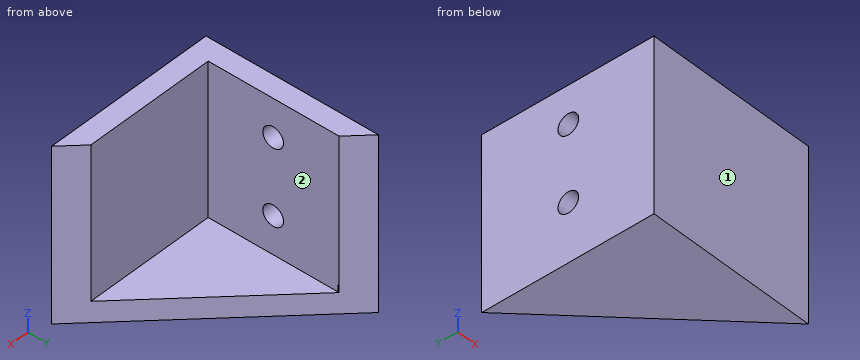
from build123d import *

# Parameters (mm, degrees)
BOSS_EXTRUDE2_DEPTH     = 25
CUT_EXTRUDE1_DEPTH      = 21
SKETCH3_W               = 26.870057685
SKETCH3_H               = 1
CUT_EXTRUDE3_DEPTH      = 0.1
CUT_EXTRUDE4_DEPTH      = 1
BOSS_EXTRUDE3_DEPTH     = 1
CUT_EXTRUDE5_DEPTH      = 15
CUT_EXTRUDE5_DEPTH_BACK = 18
SKETCH8_R               = 1.5


with BuildPart() as part:
    # Sketch1 → Boss-Extrude2 (new body)
    with BuildSketch(Plane.XY):
        Polygon((0, 24.307463671), (0, -0.692536329), (25, -0.692536329), align=None)
    extrude(amount=BOSS_EXTRUDE2_DEPTH)

    # Sketch2 → Cut-Extrude1 (cut)
    with BuildSketch(Plane.XY.offset(25)):
        Polygon((3, 21.307463671), (3, 2.307463671), (22, 2.307463671), align=None)
    extrude(amount=-CUT_EXTRUDE1_DEPTH, mode=Mode.SUBTRACT)

    # Sketch3 → Cut-Extrude3 (cut)
    with BuildSketch(Plane(origin=(12.153731836, 12.153731836, 0), x_dir=(0.7071067811865475, -0.7071067811865477, 0), z_dir=(0.7071067811865477, 0.7071067811865475, 0))):
        with Locations((0.489697135, -3.5)):
            Rectangle(SKETCH3_W, SKETCH3_H)
    extrude(amount=-CUT_EXTRUDE3_DEPTH, mode=Mode.SUBTRACT)

    # Sketch4 → Cut-Extrude4 (cut)
    with BuildSketch(Plane.XY.offset(4)):
        Polygon((3, 21.307463671), (3, 2.307463671), (22, 2.307463671), align=None)
    extrude(amount=-CUT_EXTRUDE4_DEPTH, mode=Mode.SUBTRACT)

    # Sketch5 → Boss-Extrude3 (add)
    with BuildSketch(Plane.XY.offset(3)):
        Polygon((22, 2.307463671), (21.858578644, 2.307463671), (21.929289322, 2.236752993), align=None)
    extrude(amount=BOSS_EXTRUDE3_DEPTH)

    # Sketch8 → Cut-Extrude5 (cut, two sides: drawn at the far end of the back side and taken through both)
    with BuildSketch(Plane(origin=(3, 0, 0), x_dir=(0, 0, -1), z_dir=(1, 0, 0)).offset(-CUT_EXTRUDE5_DEPTH_BACK)):
        with Locations(Location((-8.5, 11.736752993, 0), (0, 0, 270))):
            Circle(SKETCH8_R)
        with Locations(Location((-19.5, 11.736752993, 0), (0, 0, 270))):
            Circle(SKETCH8_R)
    extrude(amount=CUT_EXTRUDE5_DEPTH + CUT_EXTRUDE5_DEPTH_BACK, mode=Mode.SUBTRACT)


solid = part.part
Can you work these out from the model? Positions are in its coordinate system, mm. Face numbers are marked on the shaded views. A direction names the side the tool comes from. Give positions to 0.01 mm unless a question says otherwise; leave off trailing zeros. Loops run counter-clockwise (first coordinate to the right, second up) from the corner with the lowest first, then second, coordinate; pieces in that order, holes last. Notation, with made-up numbers: M 25.25,15 L 79.25,15 A27 cw 79.25,44 Z; hole C -1,79 d8. An arc over 180 degrees is marked long. One line per item, written item: value. Start each with the question number.
1) If we section it at A-A, the plane z = 8.5: Write out the boundary of the cut face in (x, y), and give its area (3 significant figures).
2) On a 3-axis mill with a long thin cutter (end or side, diameter ignored), from which of +Z, -Z, +X, -X, +Y, -Y can I reach the whole of each face in a straight line? I mean the marked faces 1 and 2. Say none if no direction works.
3) If we section it at C-C, the plane x = 15.5: Write out the boundary of the cut face in (y, z), and give its area (3 significant figures).
4) If we section it at B-B, the plane z = 15.75: Write out the boundary of the cut face in (x, y).
5) If I drill on line 1 (Y direction, x = 19, z = 6.5); line 2 (X direction, y = 16.25, z = 12.25), over which ranges is the centre line in solid material (lowest first)? Write a range as [from, to].
6) I'm going to push flat-ended pins straight in: pin 1 (6 mm diameter, centred on y = 7.5, z = 4, fed in from -X); pin 2 (5 mm diameter, centred on x = 11.5, z = 18.5, fed in from +Y); pin 3 (15 mm diameter, centred on y = 10, z = 14.5, fed in from +X). Where does each tip first touch, or does it pass through?
7) If we section it at D-D, the plane y = 1.5: Write out the boundary of the cut face in (x, z).
Completed:
1. outline: M 0,-0.69 L 25,-0.69 L 22,2.31 L 3,2.31 L 3,10.24 L 0,10.24 Z; M 0,13.24 L 3,13.24 L 3,21.31 L 0,24.31 Z
1. area: 123 mm^2
2. face 1: +Z, -Z, +X, -X, -Y
2. face 2: +Z, +X, +Y
3. outline: M -0.69,0 L 8.81,0 L 8.81,3 L 2.31,3 L 2.31,25 L -0.69,25 Z
3. area: 94.5 mm^2
4. outline: M 0,-0.69 L 25,-0.69 L 22,2.31 L 3,2.31 L 3,21.31 L 0,24.31 Z
5. line 1: y = [-0.69, 2.31]
5. line 2: x = [0, 3]
6. pin 1: stops at x = 0
6. pin 2: stops at y = 2.31
6. pin 3: stops at x = 3
7. outline: M 0,0 L 22.81,0 L 22.81,25 L 0,25 Z
